Input: dimensioned drawing with shaded views. Units: mm. Origin: part minimum x, y, z. A direction names the side the tool comes from. Give positions to 0.01 mm unless a question says otherwise; leave off trailing zeros. Order: outer loops, then holes, each group sorted by start corner. A loop starts at its lowest first (then second) coordinate and runs counter-clockwise, first axis right, second up.
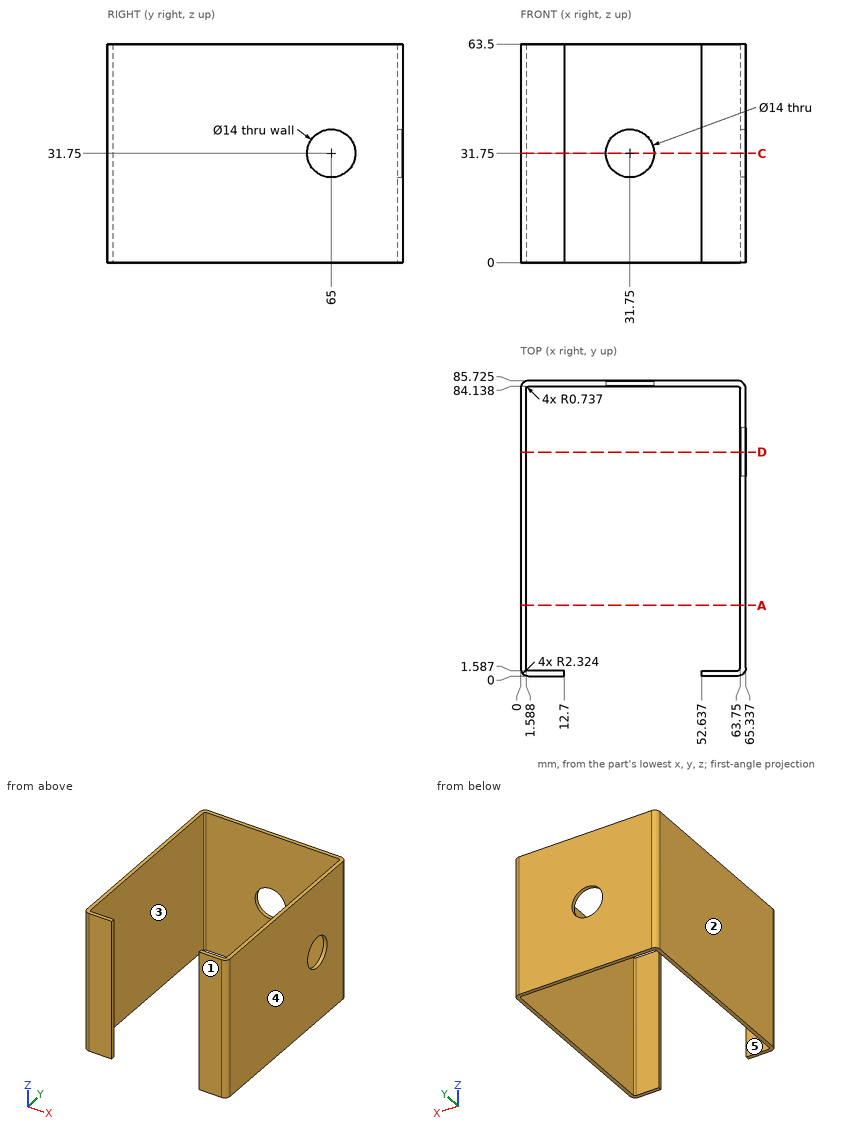
1) Pull-direction query (Y, two-part tool) for the marked faces 1, 2 and 3; classes: pulls with the +Y half, pulls with the -Y half, needs draft (parallel to the pull), parting line crosses it, or undercut.
2) Line query: probe 1 along Y at (x, z) = (4.5, 12.5) (1 decimal); probe 2 along X at (y, z) = (10, 41.5); probe 3 along Z at (x, y) = (31.75, 85.1). Output: solid intervals per line, ascending.
3) First-contact query: P1, Ø0.8, axis at y = 0.5, z = 37.5, coming from the -X side; P2, Ø0.8, axis at y = 0.5, z = 17, coming from the +X side. Flat tips, straight axial feed; report the tip coordinate or a pass-through.
4) Reachability of the marked faces 4 and 5 from +Z, -Z, +X, -X, +Y, -Y: full face, straight path, thin tool, end or side. Return the list, or none.
5) Cut plane A-A (y = 20.5). Return the cut outline in (x, z).
6) Cut plane C-C (z = 31.75). Count the separate pieces of the cut face and the enclosed holes in it.
7) Cut plane D-D (y = 65). Return the cut outline in (x, z).
Geometry says:
1. face 1: pulls with the -Y half
1. face 2: needs draft
1. face 3: undercut
2. probe 1: y = 0 to 1.6, 84.1 to 85.7
2. probe 2: x = 0 to 1.59, 63.75 to 65.34
2. probe 3: z = 0 to 24.75, 38.75 to 63.5
3. P1: stops at x = 0.49
3. P2: stops at x = 64.85
4. face 4: +Z, -Z, +X, +Y, -Y
4. face 5: +Z, -Z
5. outline: (0, 0) - (1.59, 0) - (1.59, 63.5) - (0, 63.5) - close; (63.75, 0) - (65.34, 0) - (65.34, 63.5) - (63.75, 63.5) - close
6. separate pieces: 3
6. enclosed holes: 0
7. outline: (0, 0) - (1.59, 0) - (1.59, 63.5) - (0, 63.5) - close; (63.75, 0) - (65.34, 0) - (65.34, 24.75) - (63.75, 24.75) - close; (63.75, 38.75) - (65.34, 38.75) - (65.34, 63.5) - (63.75, 63.5) - close
